```python
from build123d import *

# Parameters (mm, degrees)
SKETCH_1_R      = 1.75
EXTRUDE_1_DEPTH = 4
FILLET_1_R      = 3


with BuildPart() as part:
    # Эскиз1 → Бобышка-Вытянуть1 (new body)
    with BuildSketch(Plane.XY):
        Polygon((-27.5, -31.5), (-27.5, -45), (27.5, -45), (27.5, -31.5), (24.5, -31.5), (24.5, -32.55), (22.5, -32.55), (22.5, -31.5), (21.5, -31.5), (21.5, -28.5), (22.5, -28.5), (22.5, -27.45), (24.5, -27.45), (24.5, -28.5), (27.5, -28.5), (27.5, -15), (31.5, -15), (31.5, 15), (27.5, 15), (27.5, 10), (22.5, 10), (22.5, 17.5), (27.5, 17.5), (27.5, 21.5), (24.5, 21.5), (24.5, 20.45), (22.5, 20.45), (22.5, 21.5), (21.5, 21.5), (21.5, 24.5), (22.5, 24.5), (22.5, 25.55), (24.5, 25.55), (24.5, 24.5), (27.5, 24.5), (27.5, 45), (1.5, 45), (1.5, 42), (2.55, 42), (2.55, 40), (1.5, 40), (1.5, 39), (-1.5, 39), (-1.5, 40), (-2.55, 40), (-2.55, 42), (-1.5, 42), (-1.5, 45), (-27.5, 45), (-27.5, 31.5), (-24.5, 31.5), (-24.5, 32.55), (-22.5, 32.55), (-22.5, 31.5), (-21.5, 31.5), (-21.5, 28.5), (-22.5, 28.5), (-22.5, 27.45), (-24.5, 27.45), (-24.5, 28.5), (-27.5, 28.5), (-27.5, 15), (-31.5, 15), (-31.5, -15), (-27.5, -15), (-27.5, -28.5), (-24.5, -28.5), (-24.5, -27.45), (-22.5, -27.45), (-22.5, -28.5), (-21.5, -28.5), (-21.5, -31.5), (-22.5, -31.5), (-22.5, -32.55), (-24.5, -32.55), (-24.5, -31.5), align=None)
        with Locations((7.5, 21.1)):
            Circle(SKETCH_1_R, mode=Mode.SUBTRACT)
    extrude(amount=EXTRUDE_1_DEPTH)

    # Скругление1
    fillet_1_edges = [part.edges().sort_by_distance(p)[0] for p in [
        (22.5, 17.5, 2),
        (22.5, 10, 2),
    ]]
    fillet(fillet_1_edges, radius=FILLET_1_R)


solid = part.part
```
Design review of the part built by this model. Coordinates are the model's own, in mm. A direction names the side the tool comes from. Round coordinates to 2 decimals unless told otherwise and drop trailing zeros. Order: outer loops, then holes, each group sorted by start corner. A loop starts at its lowest first (then second) coordinate and runs counter-clockwise, first axis right, second up. Notation, with made-up numbers: M 66.5,12.25 L 101.5,12.25 A23 ccw 101.5,25.25 Z; hole C -18.75,23.5 d2. An arc over 180 degrees is marked long. Put each result on its own line as item: value.
Q1. Machinability: for faces 4 (the face through (-23, -32.55, 2)), 5 (the face through (29, -15, 2)), 6 (the face through (-26, -31.5, 2)), 7 (the face through (30, 15, 2)), 8 (the face through (26, -31.5, 2)), which of the approach directions +Z, -Z, +X, -X, +Y, -Y give a long, thin tool a straight path to every point of the face, cutting with its end or side? Answer none if there is none.
Reported:
face 4: +Z, -Z
face 5: +Z, -Z, +X, -Y
face 6: +Z, -Z, -X
face 7: +Z, -Z, +X, +Y
face 8: +Z, -Z, +X
Q2. Insertion check: pin 1 Ø2 at (x, y) = (3, 14) entering from -Z; pin 2 Ø0.5 at (y, z) = (25, 2.5) entering from +X; pin 3 Ø0.8 at (y, z) = (21, 1) entering from -X. Each pin has a flat end and moves straight along its axis. Give the tip position at first contact, or say it passes through.
Reported:
pin 1: z = 0
pin 2: x = 27.5
pin 3: x = -27.5
Q3. Consider section A-A (x = 7.5). State the section outline as (y, z) points, and give its area (3 significant figures).
Reported:
outline: M -45,0 L 19.35,0 L 19.35,4 L -45,4 Z; M 22.85,0 L 45,0 L 45,4 L 22.85,4 Z
area: 346 mm²
Q4. Draft analysis for pull direction Y (two halves, no side actions). For faces 1 (the face through (-27.5, -22, 2)), 2 (the face through (-29, 15, 2)), 3 (the face through (26, 17.5, 2)), state which applies: released by +Y, released by -Y, zero draft, split by the parting line, or undercut.
Reported:
face 1: zero draft
face 2: released by +Y
face 3: undercut
Q5. To check wall thickness, follow line 1 (Y direction, x = -27, z = 1.1); line 2 (Y direction, x = 7.5, z = 1.3); line 3 (Y direction, x = -23, z = 3). State the ranges of each line that lie inside material, in increasing order.
Reported:
line 1: -45 to -31.5, -28.5 to 28.5, 31.5 to 45
line 2: -45 to 19.35, 22.85 to 45
line 3: -45 to -32.55, -27.45 to 27.45, 32.55 to 45
